Input: part model. Units: mm. Frame: model coordinates. Face numbers are marked on the shaded views. A direction names the side the tool comes from. Give positions to 0.01 mm unless a question says otherwise; leave off trailing zeros. Write each loop counter-clockwise with the first axis right and the second up, starting at its lowest first coordinate (ties: lowest second). Pieces come first, ordered by that corner, then holes. Notation, with made-up numbers: (-36, 64.25) - (16, 64.25) arc R22 ccw to (16, 97.25) - close; hole circle Ø11 at (-25, 61.25). An arc over 180 degrees is marked (long way). Answer as CSV lines item,"result".
```python
from build123d import *

# Parameters (mm, degrees)
F0_R     = 1.5
F1_DEPTH = 3
F2_R     = 1.5
F3_DEPTH = 3


# Not quite as in the source:
# - a feature names something its author has since deleted; it is built from what else it names


with BuildPart() as f1:
    # F0 (on Front) → F1 (new body)
    with BuildSketch(Plane.XZ):
        with BuildLine():
            Line((57.5, 5), (50, 5))
            Line((50, 5), (50, 25))
            Line((50, 25), (10, 25))
            Line((10, 25), (10, 5))
            Line((10, 5), (2.5, 5))
            ThreePointArc((2.5, 5), (-2.5, 0), (2.5, -5))
            Line((2.5, -5), (57.5, -5))
            ThreePointArc((57.5, -5), (62.5, 0), (57.5, 5))
        make_face()
        with Locations((2.5, 0)):
            Circle(F0_R, mode=Mode.SUBTRACT)
        with Locations((57.5, 0)):
            Circle(F0_R, mode=Mode.SUBTRACT)
    extrude(amount=F1_DEPTH)

    # F2 (on face) → F3 (join)
    with BuildSketch(Plane.XY.offset(25)):
        Polygon((50, 0), (10, 0), (10, -3), (10, -13), (10, -23), (10, -33), (10, -43), (10, -53), (10, -63), (50, -63), (50, -53), (50, -43), (50, -33), (50, -23), (50, -13), (50, -3), align=None)
        with BuildLine():
            ThreePointArc((21.5, -53), (20, -54.5), (18.5, -53))
            ThreePointArc((18.5, -53), (20, -51.5), (21.5, -53))
        make_face(mode=Mode.SUBTRACT)
        with BuildLine():
            ThreePointArc((21.5, -43), (20, -44.5), (18.5, -43))
            ThreePointArc((18.5, -43), (20, -41.5), (21.5, -43))
        make_face(mode=Mode.SUBTRACT)
        with Locations((40, -53)):
            Circle(F2_R, mode=Mode.SUBTRACT)
        with Locations((40, -43)):
            Circle(F2_R, mode=Mode.SUBTRACT)
        with BuildLine():
            ThreePointArc((21.5, -23), (20, -24.5), (18.5, -23))
            ThreePointArc((18.5, -23), (20, -21.5), (21.5, -23))
        make_face(mode=Mode.SUBTRACT)
        with BuildLine():
            ThreePointArc((21.5, -13), (20, -14.5), (18.5, -13))
            ThreePointArc((18.5, -13), (20, -11.5), (21.5, -13))
        make_face(mode=Mode.SUBTRACT)
        with Locations((40, -23)):
            Circle(F2_R, mode=Mode.SUBTRACT)
        with Locations((40, -13)):
            Circle(F2_R, mode=Mode.SUBTRACT)
    extrude(amount=F3_DEPTH)


solid = f1.part
```
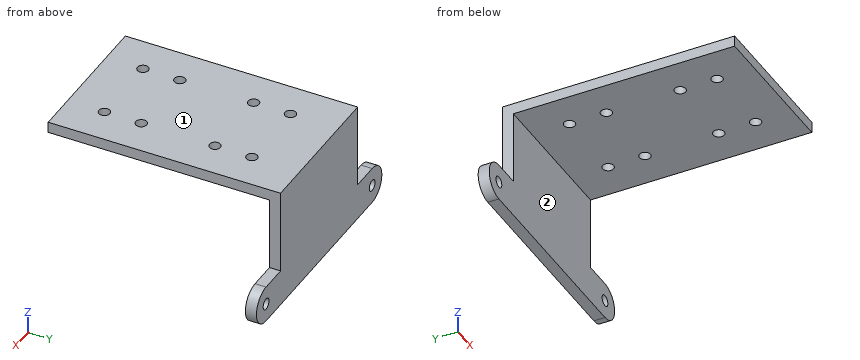
Item 1: Contact query for flat-ended pins moving along their axis: pin 1 (12 mm diameter, centred on y = -55.5, z = 24, fed in from +X); pin 2 (10 mm diameter, centred on x = 27, z = -0.5, fed in from +Y); pin 3 (3.5 mm diameter, centred on x = 40, y = -13, fed in from -Z); pin 4 (10 mm diameter, centred on x = 47, z = 4.5, fed in from -Y). Output: stop coordinate, or through.
The answers:
pin 1,"x = 50"
pin 2,"y = 0"
pin 3,"z = 25"
pin 4,"y = -3"
Item 2: Cut plane B-B on z = 0. Return the cut outline in (x, y).
The answers:
outline,"(-2.5, -3) - (1, -3) - (1, 0) - (-2.5, 0) - close; (4, -3) - (56, -3) - (56, 0) - (4, 0) - close; (59, -3) - (62.5, -3) - (62.5, 0) - (59, 0) - close"
Item 3: Cut plane D-D on z = 19. Return the cut outline in (x, y).
The answers:
outline,"(10, -3) - (50, -3) - (50, 0) - (10, 0) - close"
Item 4: Cut plane C-C on x = 20. Return the cut outline in (y, z).
The answers:
outline,"(-63, 25) - (-54.5, 25) - (-54.5, 28) - (-63, 28) - close; (-51.5, 25) - (-44.5, 25) - (-44.5, 28) - (-51.5, 28) - close; (-41.5, 25) - (-24.5, 25) - (-24.5, 28) - (-41.5, 28) - close; (-21.5, 25) - (-14.5, 25) - (-14.5, 28) - (-21.5, 28) - close; (-11.5, 25) - (-3, 25) - (-3, -5) - (0, -5) - (0, 28) - (-11.5, 28) - close"
Item 5: Ray query, line 1 (Y direction, x = 40, z = 27); line 2 (Z direction, x = 34, y = -6); line 3 (Y direction, x = 24, z = 5.5). Return the intervals inside material, ascending. Write a range as from..to.
The answers:
line 1,"-63..-54.5, -51.5..-44.5, -41.5..-24.5, -21.5..-14.5, -11.5..0"
line 2,"25..28"
line 3,"-3..0"
Item 6: Reachability of the marked faces 1 and 2 from +Z, -Z, +X, -X, +Y, -Y: full face, straight path, thin tool, end or side. Return the list, or none.
The answers:
face 1,"+Z, +X, -X, +Y, -Y"
face 2,"-Z, +X, -X, -Y"
Item 7: Cut plane A-A on y = -13. Return the cut outline in (x, z), plus the area to 3 significant figures.
The answers:
outline,"(10, 25) - (18.5, 25) - (18.5, 28) - (10, 28) - close; (21.5, 25) - (38.5, 25) - (38.5, 28) - (21.5, 28) - close; (41.5, 25) - (50, 25) - (50, 28) - (41.5, 28) - close"
area,"102 mm²"
